```python
from build123d import *

# Parameters (mm, degrees)
F0_R     = 34.8107
F1_DEPTH = 25.146
F2_R     = 3.4798
F3_R     = 0.635
F6_R     = 1.27


with BuildPart() as f1:
    # F0 (on Top) → F1 (new body)
    with BuildSketch(Plane.XY):
        Circle(F0_R)
    extrude(amount=F1_DEPTH)

    # F2
    f2_edges = [f1.edges().sort_by_distance(p)[0] for p in [
        (-34.8107, 0, 25.146),
    ]]
    fillet(f2_edges, radius=F2_R)

    # F3
    f3_edges = [f1.edges().sort_by_distance(p)[0] for p in [
        (-34.8107, 0, 0),
    ]]
    fillet(f3_edges, radius=F3_R)

    # F4 (on Front) → F5 (revolve, cut)
    with BuildSketch(Plane.XZ):
        with BuildLine():
            Line((0, 25.146), (0, 24.1046))
            Line((0, 24.1046), (30.2895, 24.1046))
            ThreePointArc((30.2895, 24.1046), (30.594519, 24.840981), (31.3309, 25.146))
            Line((31.3309, 25.146), (0, 25.146))
        make_face()
    revolve(axis=Axis((0, 0, 24.6253), (0, 0, 1)), mode=Mode.SUBTRACT)

    # F6
    f6_edges = [f1.edges().sort_by_distance(p)[0] for p in [
        (-30.2895, 0, 24.1046),
    ]]
    fillet(f6_edges, radius=F6_R)


solid = f1.part
```
Source: CAD feature listing. Evaluate the final solid. Frame: model axes, mm. Round coordinates to 2 decimals unless told otherwise and drop trailing zeros. Loops run counter-clockwise (first coordinate to the right, second up) from the corner with the lowest first, then second, coordinate; pieces in that order, holes last.
(1) Contact query for flat-ended pins moving along their axis: pin 1 Ø1 at (y, z) = (-26, 2.5) entering from -X; pin 2 Ø1.5 at (y, z) = (3.5, 20) entering from +X; pin 3 Ø1 at (x, y) = (27, -12.5) entering from -Z; pin 4 Ø5 at (y, z) = (-4.5, 21) entering from +X. Output: stop coordinate, or through.
From the geometry:
pin 1: stops at x = -23.7
pin 2: stops at x = 34.7
pin 3: stops at z = 0
pin 4: stops at x = 34.75
(2) Section query A-A (z = 14.75). Output: boundary loops of the cut face in (x, y).
From the geometry:
outline: circle Ø69.62 at (0, 0)
(3) Material intervals for probe 1 along Z at (x, y) = (-15.5, -11.5); probe 2 along Z at (x, y) = (-11.5, 29); probe 3 along X at (y, z) = (-28, 22), sorted ascending.
From the geometry:
probe 1: z = 0 to 24.1
probe 2: z = 0 to 25.14
probe 3: x = -20.66 to 20.66
(4) Pull-direction query (Y, two-part tool) for faces 1 (the flat face through (0, 0, 24.105)), 2 (the flat face through (0, 0, 0)), 3 (the cylindrical face through (-4.532, 34.514, 11.003)); classes: +Y half, -Y half, draft (parallel to the pull), parting line (faces both ways), or undercut.
From the geometry:
face 1: undercut
face 2: draft
face 3: parting line
